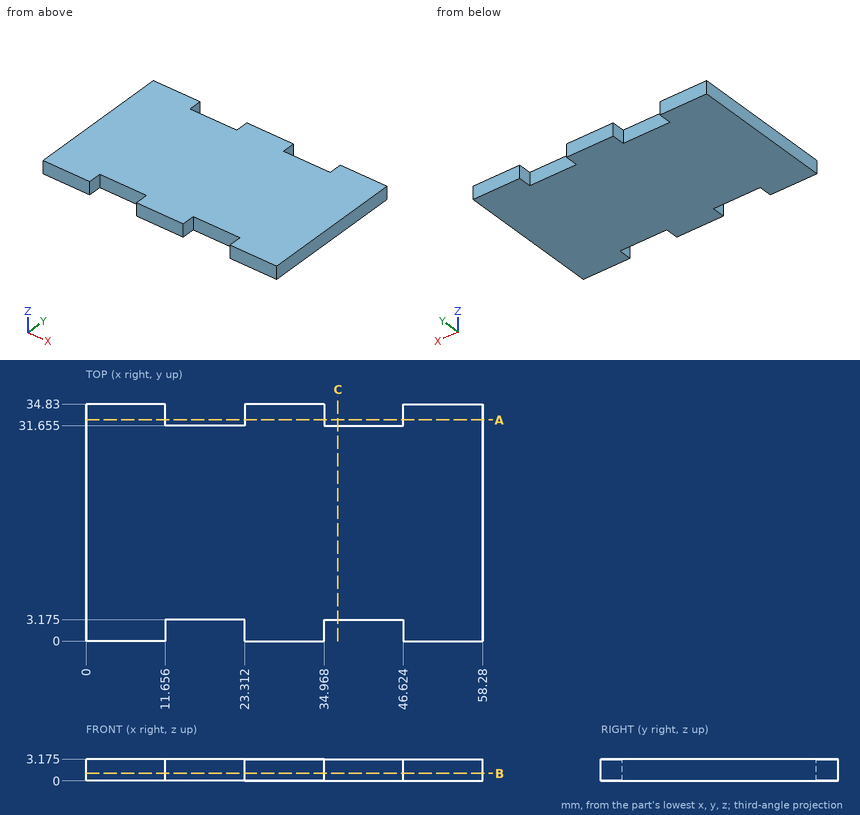
Can you work these out from the drawing? Everything is in mm from the part's minimum corner. Round coordinates to 2 decimals unless told otherwise and drop trailing zeros. Loops run counter-clockwise (first coordinate to the right, second up) from the corner with the lowest first, then second, coordinate; pieces in that order, holes last. Notation, with made-up numbers: (25.5, -29) - (64.5, -29) arc R19 ccw to (64.5, -13) - close; hole circle Ø9 at (85, -6.5). An arc over 180 degrees is marked (long way). Write item = value, one per line. Start each with the question number.
(1) For P1, Ø1, axis at x = 38.5, z = 1.5, coming from the -Y side (3 decimals); P2, Ø1, axis at x = 14.5, z = 2.5, coming from the +Y side (3 decimals), each with a flat end and sliding along its axis, tell me the tip position at first contact or that it passes through.
(2) If we section it at C-C (x = 37): Please give me the cut outline in (y, z) (3 decimals), and give its area (3 significant figures).
(3) If I drill on probe 1 along X at (y, z) = (2, 1); probe 2 along Y at (x, z) = (41.5, 0.65) (3 decimals), over which ranges is the centre line in solid material (lowest first)? Write a range as [from, to].
(4) If we section it at B-B (z = 1.1): Please give me the cut outline in (x, y) (3 decimals), and give its area (3 significant figures).
(5) If we section it at A-A (y = 32.5): Please give me the cut outline in (x, z) (3 decimals).
Ans:
q1.P1 = 3.175
q1.P2 = 31.655
q2.outline = (3.175, 0) - (31.655, 0) - (31.655, 3.175) - (3.175, 3.175) - close
q2.area = 90.4 mm²
q3.probe_1 = [0, 11.66], [23.31, 34.97], [46.62, 58.28]
q3.probe_2 = [3.175, 31.655]
q4.outline = (0, 0) - (11.656, 0) - (11.656, 3.175) - (23.312, 3.175) - (23.312, 0) - (34.968, 0) - (34.968, 3.175) - (46.624, 3.175) - (46.624, 0) - (58.28, 0) - (58.28, 34.83) - (46.624, 34.83) - (46.624, 31.655) - (34.968, 31.655) - (34.968, 34.83) - (23.312, 34.83) - (23.312, 31.655) - (11.656, 31.655) - (11.656, 34.83) - (0, 34.83) - close
q4.area = 1,880 mm²
q5.outline = (0, 0) - (11.656, 0) - (11.656, 3.175) - (0, 3.175) - close; (23.312, 0) - (34.968, 0) - (34.968, 3.175) - (23.312, 3.175) - close; (46.624, 0) - (58.28, 0) - (58.28, 3.175) - (46.624, 3.175) - close
